CAD build for the part. Positions are in the model's coordinates, mm. Face numbers are marked on the shaded views. Round coordinates to 2 decimals unless told otherwise and drop trailing zeros. Order: outer loops, then holes, each group sorted by start corner. A loop starts at its lowest first (then second) coordinate and runs counter-clockwise, first axis right, second up. Notation, with made-up numbers: (53, 61.25) - (92, 61.25) arc R20 ccw to (92, 99.25) - close; hole circle Ø4 at (36.5, 3). An arc over 180 degrees is marked (long way). Write item = value, one per line.
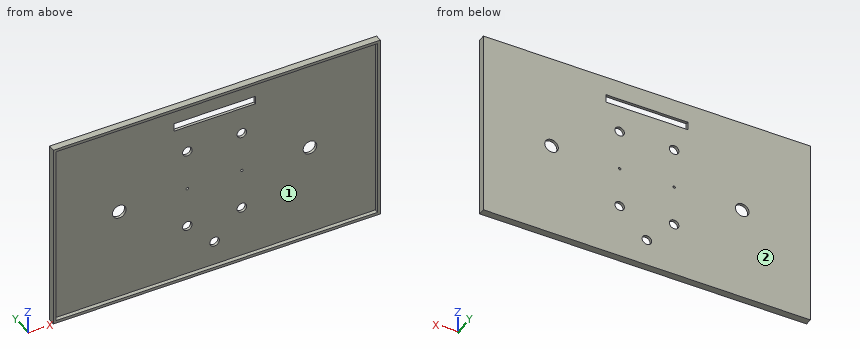
from build123d import *

# Parameters (mm, degrees)
SKETCH1_W                 = 304.8
SKETCH1_H                 = 177.8
BOSS_EXTRUDE1_DEPTH       = 101.6
SHELL1_T                  = 2.54
SKETCH3_R                 = 6.35
CUT_EXTRUDE1_DEPTH        = 2.54
F_4_40_TAPPED_HOLE1_D     = 2.2606
F_4_40_TAPPED_HOLE1_DEPTH = 2.54
SKETCH11_R                = 4.445
CUT_EXTRUDE2_DEPTH        = 2.54
SKETCH12_R                = 4.445
SKETCH12_W                = 76.2
SKETCH12_H                = 7.62
CUT_EXTRUDE3_DEPTH        = 2.54
SKETCH13_R                = 10.659380334
CUT_EXTRUDE4_DEPTH        = 2.54
SKETCH14_W                = 177.8
SKETCH14_H                = 95.25
CUT_EXTRUDE5_DEPTH        = 334.35988061


with BuildPart() as part:
    # Sketch1 → Boss-Extrude1 (new body)
    with BuildSketch(Plane(origin=(0, 0, 0), x_dir=(1, 0, 0), z_dir=(0, 1, 0))):
        Rectangle(SKETCH1_W, SKETCH1_H)
    extrude(amount=BOSS_EXTRUDE1_DEPTH)

    # Shell1 (no face opened: a closed hollow body)
    add(offset(amount=-SHELL1_T, mode=Mode.PRIVATE), mode=Mode.SUBTRACT)

    # Sketch3 → Cut-Extrude1 (cut)
    with BuildSketch(Plane(origin=(0, 101.6, 0), x_dir=(1, 0, 0), z_dir=(0, 1, 0))):
        with Locations(Location((-88.9, 0, 0), (0, 0, 270))):
            Circle(SKETCH3_R)
        with Locations(Location((88.9, 0, 0), (0, 0, 270))):
            Circle(SKETCH3_R)
    extrude(amount=-CUT_EXTRUDE1_DEPTH, mode=Mode.SUBTRACT)

    # #4-40 Tapped Hole1
    with Locations(Plane(origin=(0, 101.6, 0), x_dir=(1, 0, 0), z_dir=(0, 1, 0))):
        with Locations((-25.4, 0), (25.4, 0)):
            Hole(F_4_40_TAPPED_HOLE1_D / 2, depth=F_4_40_TAPPED_HOLE1_DEPTH)

    # Sketch11 → Cut-Extrude2 (cut)
    with BuildSketch(Plane(origin=(0, 101.6, 0), x_dir=(1, 0, 0), z_dir=(0, 1, 0))):
        with Locations(Location((-25.4, 38.1, 0), (0, 0, 270))):
            Circle(SKETCH11_R)
        with Locations(Location((25.4, 38.1, 0), (0, 0, 270))):
            Circle(SKETCH11_R)
        with Locations(Location((25.4, -38.1, 0), (0, 0, 270))):
            Circle(SKETCH11_R)
        with Locations(Location((-25.4, -38.1, 0), (0, 0, 270))):
            Circle(SKETCH11_R)
    extrude(amount=-CUT_EXTRUDE2_DEPTH, mode=Mode.SUBTRACT)

    # Sketch12 → Cut-Extrude3 (cut)
    with BuildSketch(Plane(origin=(0, 101.6, 0), x_dir=(1, 0, 0), z_dir=(0, 1, 0))):
        with Locations(Location((0, 63.5, 0), (0, 0, 270))):
            Circle(SKETCH12_R)
        with Locations((0, -67.31)):
            Rectangle(SKETCH12_W, SKETCH12_H)
    extrude(amount=-CUT_EXTRUDE3_DEPTH, mode=Mode.SUBTRACT)

    # Sketch13 → Cut-Extrude4 (cut)
    with BuildSketch(Plane.XY.offset(88.9)):
        with Locations((0, 50.8)):
            Circle(SKETCH13_R)
    extrude(amount=-CUT_EXTRUDE4_DEPTH, mode=Mode.SUBTRACT)

    # Sketch14 → Cut-Extrude5 (cut, through all)
    with BuildSketch(Plane.ZY.offset(152.4)):
        with Locations((0, 47.625)):
            Rectangle(SKETCH14_W, SKETCH14_H)
    extrude(amount=-CUT_EXTRUDE5_DEPTH, mode=Mode.SUBTRACT)


solid = part.part
(1) Drop flat-ended pins along their axis: pin 1 (4 mm diameter, centred on x = -97, z = 63.5, fed in from -Y); pin 2 (7 mm diameter, centred on x = 0, z = -63.5, fed in from +Y). Give the stop position or say it passes through.
Solved:
pin_1 = 99.06
pin_2 = through
(2) Band-saw the part on C-C on z = -38.1. List the corners of the cut face in (x, y) (3 decimals), plus the area to 3 significant figures.
Solved:
outline = (-152.4, 95.25) - (-149.86, 95.25) - (-149.86, 99.06) - (-29.845, 99.06) - (-29.845, 101.6) - (-152.4, 101.6) - close; (-20.955, 99.06) - (20.955, 99.06) - (20.955, 101.6) - (-20.955, 101.6) - close; (29.845, 99.06) - (149.86, 99.06) - (149.86, 95.25) - (152.4, 95.25) - (152.4, 101.6) - (29.845, 101.6) - close
area = 748 mm²
(3) Pull direction Z, two halves, no side cores. Call the marked faces 1 and 2: released by +Z, released by -Z, zero draft, split by the parting line, or undercut.
Solved:
face_1 = undercut
face_2 = zero draft
(4) Probe line 1 along X through (y, z) = (101.25, 38.5); line 2 along Z through (x, y) = (99, 97); line 3 along X through (y, z) = (97.25, 20). List the from-to ranges inside material, lowest first.
Solved:
line_1 = -152.4 to -29.83, -20.97 to 20.97, 29.83 to 152.4
line_2 = -88.9 to -86.36, 86.36 to 88.9
line_3 = -152.4 to -149.86, 149.86 to 152.4
(5) Band-saw the part on A-A on x = 0. List the corners of the cut face in (y, z) (3 decimals).
Solved:
outline = (95.25, -88.9) - (101.6, -88.9) - (101.6, -67.945) - (99.06, -67.945) - (99.06, -86.36) - (95.25, -86.36) - close; (95.25, 86.36) - (99.06, 86.36) - (99.06, 71.12) - (101.6, 71.12) - (101.6, 88.9) - (95.25, 88.9) - close; (99.06, -59.055) - (101.6, -59.055) - (101.6, 63.5) - (99.06, 63.5) - close
(6) Band-saw the part on B-B on y = 97.5. List the corners of the cut face in (x, z).
Solved:
outline = (-152.4, -88.9) - (152.4, -88.9) - (152.4, 88.9) - (-152.4, 88.9) - close; hole (-149.86, -86.36) - (149.86, -86.36) - (149.86, 86.36) - (-149.86, 86.36) - close
(7) Band-saw the part on D-D on x = 88.9. List the corners of the cut face in (y, z).
Solved:
outline = (95.25, -88.9) - (101.6, -88.9) - (101.6, -6.35) - (99.06, -6.35) - (99.06, -86.36) - (95.25, -86.36) - close; (95.25, 86.36) - (99.06, 86.36) - (99.06, 6.35) - (101.6, 6.35) - (101.6, 88.9) - (95.25, 88.9) - close
